Input: part model. Units: mm. Frame: model coordinates. Give positions to 0.01 mm unless a question says otherwise; leave off trailing zeros. Loops run counter-clockwise (first coordinate to the right, second up) from the corner with the lowest first, then second, coordinate; pieces in that order, holes last. Notation, with made-up numbers: M 53.5,34.5 L 108.5,34.5 A23 cw 108.5,65.5 Z; hole C 48.5,67.25 d11. An arc over 180 degrees is marked long. Use a Markdown table: item, result. Add a question column.
from build123d import *

# Parameters (mm, degrees)
F0_R     = 4.199999
F0_R_2   = 3.300001
F0_W     = 5.2
F0_H     = 6.199998
F1_DEPTH = 2


# Not quite as in the source:
# - ends of sketch curves that miss each other by under 0.0002 mm in the source are joined


with BuildPart() as f1:
    # F0 (on Front) → F1 (new body)
    with BuildSketch(Plane.XZ):
        Polygon((-35.399994, -61.250012), (-35.399994, -64.250012), (35.399993, -64.250012), (35.399993, 64.250001), (25.199994, 64.250011), (15.100006, 64.250011), (-35.399994, 64.250011), align=None)
        with BuildLine():
            Line((-28.699995, -62.750012), (-29.599993, -62.750012))
            ThreePointArc((-29.599993, -62.750012), (-30.199994, -61.2500123621), (-29.5999938002, -59.7500141903))
            Line((-29.5999938002, -59.7500141903), (-28.699995, -59.750013))
            ThreePointArc((-28.699995, -59.750013), (-27.8999944412, -59.550011), (-27.099993, -59.750013))
            Line((-27.099993, -59.750013), (-26.199995, -59.750013))
            ThreePointArc((-26.199995, -59.750013), (-25.599994, -61.2500123621), (-26.1999951748, -62.7500108335))
            Line((-26.1999951748, -62.7500108335), (-27.099993, -62.750012))
            ThreePointArc((-27.099993, -62.750012), (-27.8999944412, -62.950014), (-28.699995, -62.750012))
        make_face(mode=Mode.SUBTRACT)
        with Locations((-25.400037, -47.249964)):
            Circle(F0_R, mode=Mode.SUBTRACT)
        with Locations((-25.400037, -32.249966)):
            Circle(F0_R, mode=Mode.SUBTRACT)
        with Locations((-12.700012, -47.249939)):
            Circle(F0_R, mode=Mode.SUBTRACT)
        with Locations((-12.700063, -32.249938)):
            Circle(F0_R, mode=Mode.SUBTRACT)
        with Locations((-3.7e-05, -47.249964)):
            Circle(F0_R, mode=Mode.SUBTRACT)
        with Locations((-23.400008, -8.750001)):
            Circle(F0_R_2, mode=Mode.SUBTRACT)
        with Locations((12.699963, -47.249964)):
            Circle(F0_R, mode=Mode.SUBTRACT)
        with BuildLine():
            ThreePointArc((27.179992, -59.75), (27.9799934412, -59.549998), (28.7799947785, -59.7500004152))
            Line((28.7799947785, -59.7500004152), (29.679992, -59.75))
            ThreePointArc((29.679992, -59.75), (30.279993, -61.25), (29.6799923008, -62.7499983341))
            Line((29.6799923008, -62.7499983341), (28.779994, -62.749999))
            ThreePointArc((28.779994, -62.749999), (27.9799934412, -62.950001), (27.179992, -62.749999))
            Line((27.179992, -62.749999), (26.279994, -62.749999))
            ThreePointArc((26.279994, -62.749999), (25.679993, -61.25), (26.2799941748, -59.7500011665))
            Line((26.2799941748, -59.7500011665), (27.179992, -59.75))
        make_face(mode=Mode.SUBTRACT)
        with Locations((25.400013, -47.249921)):
            Circle(F0_R, mode=Mode.SUBTRACT)
        with Locations((3.969993, -23.379999)):
            Circle(F0_R_2, mode=Mode.SUBTRACT)
        with Locations((23.019993, -23.379999)):
            Circle(F0_R_2, mode=Mode.SUBTRACT)
        with Locations((21.74983, -5.600162)):
            Rectangle(F0_W, F0_H, mode=Mode.SUBTRACT)
        with Locations((-23.400008, 16.25)):
            Circle(F0_R_2, mode=Mode.SUBTRACT)
        with Locations((-23.400008, 41.250001)):
            Circle(F0_R_2, mode=Mode.SUBTRACT)
        with BuildLine():
            Line((-28.700008, 59.750002), (-29.600006, 59.750002))
            ThreePointArc((-29.600006, 59.750002), (-30.200007, 61.250002), (-29.6000038751, 62.7500028811))
            Line((-29.6000038751, 62.7500028811), (-28.700008, 62.750001))
            ThreePointArc((-28.700008, 62.750001), (-27.9000065588, 62.950003), (-27.1000052215, 62.7500005848))
            Line((-27.1000052215, 62.7500005848), (-26.200008, 62.750001))
            ThreePointArc((-26.200008, 62.750001), (-25.600007, 61.250002), (-26.2000076992, 59.7500036659))
            Line((-26.2000076992, 59.7500036659), (-27.100006, 59.750002))
            ThreePointArc((-27.100006, 59.750002), (-27.9000065588, 59.55), (-28.700008, 59.750002))
        make_face(mode=Mode.SUBTRACT)
        with Locations((6.268744, 6.048941)):
            Circle(F0_R_2, mode=Mode.SUBTRACT)
        with Locations((15.399993, 37.580001)):
            Circle(F0_R_2, mode=Mode.SUBTRACT)
        with BuildLine():
            Line((27.179992, 59.750025), (26.279994, 59.750025))
            ThreePointArc((26.279994, 59.750025), (25.679993, 61.2500246379), (26.2799936754, 62.7500233092))
            Line((26.2799936754, 62.7500233092), (27.179992, 62.750024))
            ThreePointArc((27.179992, 62.750024), (27.9799934412, 62.950026), (28.7799947785, 62.7500235848))
            Line((28.7799947785, 62.7500235848), (29.679992, 62.750024))
            ThreePointArc((29.679992, 62.750024), (30.279993, 61.2500246379), (29.6799923008, 59.7500266659))
            Line((29.6799923008, 59.7500266659), (28.779994, 59.750025))
            ThreePointArc((28.779994, 59.750025), (27.9799934412, 59.550023), (27.179992, 59.750025))
        make_face(mode=Mode.SUBTRACT)
    extrude(amount=F1_DEPTH)


solid = f1.part
1) Section query B-B, the plane x = 23. Return the cut outline in (y, z), and give its area (3 significant figures).
2) Section query C-C, the plane z = -45. Return the cut outline in (x, y).
3) Section query D-D, the plane y = -1.4. State how many separate pieces and enclosed holes the cut face has, and give its area (3 significant figures).
4) Pull-direction query (Z, two-part tool) for faces 1 (the flat face through (0, 0, 1)), 2 (the cylindrical face through (-20.25, -0.99, -7.76)), 3 (the cylindrical face through (16.92, -0.99, 34.65)); classes: pulls with the +Z half, pulls with the -Z half, needs draft (parallel to the pull), parting line crosses it, or undercut.
5) Ray query, line 1 (X direction, y = -1.05, z = -8.75); line 2 (Z direction, x = -9, y = -0.8); line 3 (X direction, y = -1.8, z = -4). Return the intervals inside material, ascending. Write a range as [from, to].
6) Section query A-A, the plane z = 16.25. Return the cut outline in (x, y).
Entries:
| question | item | result |
|---|---|---|
| 1 | outline | M -2,-64.25 L 0,-64.25 L 0,-50.7 L -2,-50.7 Z; M -2,-43.8 L 0,-43.8 L 0,-26.68 L -2,-26.68 Z; M -2,-20.08 L 0,-20.08 L 0,-8.7 L -2,-8.7 Z; M -2,-2.5 L 0,-2.5 L 0,64.25 L -2,64.25 Z |
| 1 | area | 218 mm² |
| 2 | outline | M -35.4,-2 L -28.95,-2 L -28.95,0 L -35.4,0 Z; M -21.85,-2 L -16.25,-2 L -16.25,0 L -21.85,0 Z; M -9.15,-2 L -3.55,-2 L -3.55,0 L -9.15,0 Z; M 3.55,-2 L 9.15,-2 L 9.15,0 L 3.55,0 Z; M 16.25,-2 L 21.85,-2 L 21.85,0 L 16.25,0 Z; M 28.95,-2 L 35.4,-2 L 35.4,0 L 28.95,0 Z |
| 3 | separate pieces | 1 |
| 3 | enclosed holes | 19 |
| 3 | area | 8,390 mm² |
| 4 | face 1 | needs draft |
| 4 | face 2 | undercut |
| 4 | face 3 | undercut |
| 5 | line 1 | x = [-35.4, -26.7], [-20.1, 35.4] |
| 5 | line 2 | z = [-64.25, -49.24], [-45.26, -34.24], [-30.26, 64.25] |
| 5 | line 3 | x = [-35.4, 19.15], [24.35, 35.4] |
| 6 | outline | M -35.4,-2 L -26.7,-2 L -26.7,0 L -35.4,0 Z; M -20.1,-2 L 35.4,-2 L 35.4,0 L -20.1,0 Z |
